from build123d import *

# Parameters (mm, degrees)
PAD_DEPTH        = 20
POCKET_DEPTH     = 25.001
HOLE_D           = 3.4
HOLE_DEPTH       = 25
HOLE_CSINK_D     = 6.7
HOLE_CSINK_ANGLE = 90
SKETCH029_R      = 1.25
HOLE002_DEPTH    = 3.001
CHAMFER003_SIZE  = 4


with BuildPart() as part:
    # Sketch → Pad (new body)
    with BuildSketch(Plane.XY):
        Polygon((0, 0), (0, 25), (-3, 25), (-3, 3), (-15, 3), (-15, 0), align=None)
    extrude(amount=PAD_DEPTH)

    # Sketch027 → Pocket (cut, through all)
    with BuildSketch(Plane.XZ):
        with BuildLine():
            Line((-3, 20), (-5.811082, 14))
            ThreePointArc((-5.811082, 14), (-5.952199, 13.58613), (-6, 13.151483))
            Line((-6, 13.151483), (-6, 10))
            ThreePointArc((-10, 10), (-8, 8), (-6, 10))
            Line((-10, 10), (-10, 12))
            ThreePointArc((-10, 12), (-10.585786, 13.414214), (-12, 14))
            Line((-12, 14), (-13, 14))
            ThreePointArc((-13, 14), (-14.414214, 13.414214), (-15, 12))
            Line((-15, 12), (-15, 20))
            Line((-15, 20), (-3, 20))
        make_face()
    extrude(amount=-POCKET_DEPTH, mode=Mode.SUBTRACT)

    # Hole
    with Locations(Plane(origin=(-3, 0, 0), x_dir=(0, 1, 0), z_dir=(-1, 0, 0))):
        with Locations((10, -5)):
            CounterSinkHole(HOLE_D / 2, HOLE_CSINK_D / 2, depth=HOLE_DEPTH, counter_sink_angle=HOLE_CSINK_ANGLE)

    # Sketch029 → Hole002 (cut, through all)
    with BuildSketch(Plane.YZ.offset(-3)):
        with Locations((20, 15)):
            Circle(SKETCH029_R)
    extrude(amount=HOLE002_DEPTH, mode=Mode.SUBTRACT)

    # Chamfer003
    chamfer003_edges = [part.edges().sort_by_distance(p)[0] for p in [
        (-15, 1.5, 0),
        (-1.5, 25, 0),
        (-1.5, 25, 20),
    ]]
    chamfer(chamfer003_edges, length=CHAMFER003_SIZE)


solid = part.part
Design review of the part built by this model. Coordinates are the model's own, in mm. A direction names the side the tool comes from. Give positions to 0.01 mm unless a question says otherwise; leave off trailing zeros. Loops run counter-clockwise (first coordinate to the right, second up) from the corner with the lowest first, then second, coordinate; pieces in that order, holes last. Notation, with made-up numbers: M 41,-15 L 86,-15 A27 cw 86,18 Z; hole C -15.5,64 d11. An arc over 180 degrees is marked long. Answer as a JSON object with one key per item and string values.
Item 1: For P1, Ø6, axis at x = -7.5, z = 10, coming from the +Y side; P2, Ø1.5, axis at x = -13.5, z = 15, coming from the -Y side; P3, Ø1.1, axis at x = -12.5, y = 1.5, coming from the +Z side; P4, Ø0.6, axis at y = 2, z = 11, coming from the +X side, all flat-tipped, find the tip position at first contact; note any pin that passes through.
Output values:
{"P1": "stops at y = 3", "P2": "passes through", "P3": "stops at z = 14", "P4": "stops at x = 0"}
Item 2: We need section D-D (z = 5). State the section outline as (x, y) points, and give its area (3 significant figures).
Output values:
{"outline": "M -15,0 L 0,0 L 0,8.3 L -1.35,8.3 L -3,6.65 L -3,3 L -15,3 Z; M -3,13.35 L -1.35,11.7 L 0,11.7 L 0,25 L -3,25 Z", "area": "98.1 mm2"}
Item 3: Wall thickness on line 1 along Z through (x, y) = (-0.55, 10); line 2 along Z through (x, y) = (-1.9, 20); line 3 along Y through (x, z) = (-1.9, 15): over which ranges is each line inside the solid? List them lowest first.
Output values:
{"line 1": "z = 0 to 3.3, 6.7 to 20", "line 2": "z = 0 to 13.75, 16.25 to 20", "line 3": "y = 0 to 18.75, 21.25 to 25"}
Item 4: Machinability: for faces 1 (the face through (-12.5, 1.5, 14)), 2 (the face through (-9, 3, 8)), 3 (the face through (-1, 23, 2)), 4 (the face through (-6, 0, 8)), 5 (the face through (-6, 1, 12)), which of the approach directions +Z, -Z, +X, -X, +Y, -Y give a long, thin tool a straight path to every point of the face, cutting with its end or side? Answer none if there is none.
Output values:
{"face 1": "+Z, -X, +Y, -Y", "face 2": "+Z, -Z, -X, +Y", "face 3": "-Z, +X, -X, +Y", "face 4": "+Z, -Z, +X, -X, -Y", "face 5": "+Z, +Y, -Y"}
Item 5: Mouldability with a two-part tool opening along Z and no side actions: class faces 6 (the face through (-5.95, 1.48, 13.59)), 7 (the face through (-0.7, 9.2, 6.5)), 8 (the face through (-13, 2, 2)) as pulls with the +Z half, pulls with the -Z half, needs draft (parallel to the pull), parting line crosses it, or undercut.
Output values:
{"face 6": "pulls with the +Z half", "face 7": "undercut", "face 8": "pulls with the -Z half"}
Item 6: We need section B-B (y = 10). State the section outline as (x, z) points.
Output values:
{"outline": "M -3,0 L 0,0 L 0,3.3 L -1.35,3.3 L -3,1.65 Z; M -3,8.35 L -1.35,6.7 L 0,6.7 L 0,20 L -3,20 Z"}
Item 7: We need section A-A (z = 11). State the section outline as (x, y) points, and give its area (3 significant figures).
Output values:
{"outline": "M -15,0 L -10,0 L -10,3 L -15,3 Z; M -6,0 L 0,0 L 0,25 L -3,25 L -3,3 L -6,3 Z", "area": "99.0 mm2"}
Item 8: We need section C-C (x = -1). State the section outline as (y, z) points, and give its area (3 significant figures).
Output values:
{"outline": "M 0,0 L 21,0 L 25,4 L 25,16 L 21,20 L 0,20 Z; hole C 10,5 d3.4; hole C 20,15 d2.5", "area": "470 mm2"}
